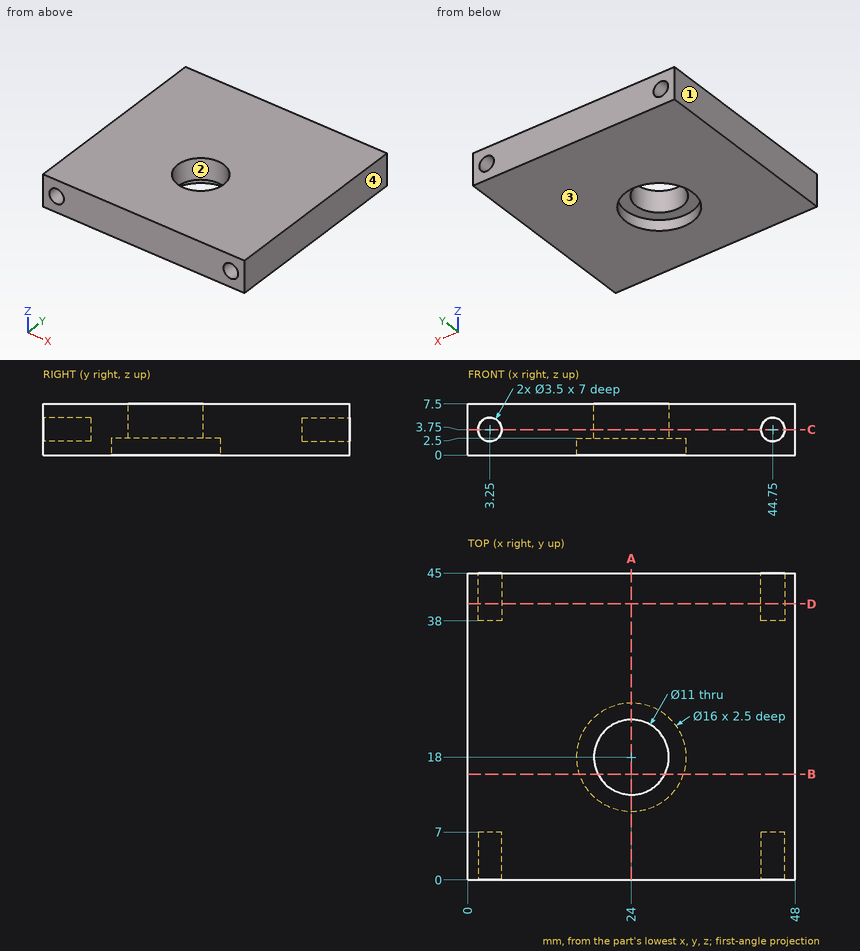
Could you check a few things on this drawing? It's one solid part, dimensions in mm from its lowest x, y, z. Round coordinates to 2 decimals unless told otherwise and drop trailing zeros. Write each loop counter-clockwise with the first axis right and the second up, starting at its lowest first coordinate (ties: lowest second). Pieces come first, ordered by that corner, then holes.
Q1. If we section it at C-C on z = 3.75: Write out the boundary of the cut face in (x, y).
Q2. If we section it at B-B on y = 15.5: Write out the boundary of the cut face in (x, z).
Q3. Will these pins go through, and if not, where does the flat tip stop? P1, Ø3, axis at x = 3.25, z = 3.75, coming from the -Y side; P2, Ø3, axis at x = 44.75, z = 3.75, coming from the +Y side.
Q4. If we section it at A-A on x = 24: Write out the boundary of the cut face in (y, z).
Q5. If we mould it in two halves opening along X, with no side actions, what happens to the marked faces 1, 2, 3 and 4? For each: +X half, -X half, draft (parallel to the pull), parting line (faces both ways), or undercut.
Q6. Please list where these lines run through material, in increasing order: probe 1 along X at (y, z) = (42.75, 3.75); probe 2 along X at (y, z) = (40.5, 5.25); probe 3 along Z at (x, y) = (44.75, 4.25).
Q7. If we section it at D-D on y = 40.5: Write out the boundary of the cut face in (x, z).
Answer below:
1. outline: (0, 0) - (1.5, 0) - (1.5, 7) - (5, 7) - (5, 0) - (43, 0) - (43, 7) - (46.5, 7) - (46.5, 0) - (48, 0) - (48, 45) - (46.5, 45) - (46.5, 38) - (43, 38) - (43, 45) - (5, 45) - (5, 38) - (1.5, 38) - (1.5, 45) - (0, 45) - close; hole circle Ø11 at (24, 18)
2. outline: (0, 0) - (16.4, 0) - (16.4, 2.5) - (19.1, 2.5) - (19.1, 7.5) - (0, 7.5) - close; (28.9, 2.5) - (31.6, 2.5) - (31.6, 0) - (48, 0) - (48, 7.5) - (28.9, 7.5) - close
3. P1: stops at y = 7
3. P2: stops at y = 38
4. outline: (0, 0) - (10, 0) - (10, 2.5) - (12.5, 2.5) - (12.5, 7.5) - (0, 7.5) - close; (23.5, 2.5) - (26, 2.5) - (26, 0) - (45, 0) - (45, 7.5) - (23.5, 7.5) - close
5. face 1: -X half
5. face 2: undercut
5. face 3: draft
5. face 4: +X half
6. probe 1: x = 0 to 1.5, 5 to 43, 46.5 to 48
6. probe 2: x = 0 to 2.35, 4.15 to 43.85, 45.65 to 48
6. probe 3: z = 0 to 2, 5.5 to 7.5
7. outline: (0, 0) - (48, 0) - (48, 7.5) - (0, 7.5) - close; hole circle Ø3.5 at (3.25, 3.75); hole circle Ø3.5 at (44.75, 3.75)
